Could you check a few things on this model? Use its own coordinates, in mm. Face numbers are marked on the shaded views. A direction names the side the tool comes from. Give positions to 0.01 mm unless a question says otherwise; leave off trailing zeros. Order: outer loops, then holes, each group sorted by start corner. A loop starts at its lowest first (then second) coordinate and runs counter-clockwise, first axis right, second up. Notation, with made-up numbers: M 75.25,-32.5 L 129.25,-32.5 A28 ccw 129.25,2.5 Z; hole C 65,-7.5 d11. An arc over 180 degrees is marked long. Use a Markdown table: item, result. Add a question column.
```python
from build123d import *

# Parameters (mm, degrees)
F0_R          = 5
F1_DEPTH      = 10.1
F2_R          = 4.8
F3_DEPTH      = 3
F5_DEPTH      = 5
F5_DEPTH_BACK = 68
F6_R          = 6
F7_DEPTH      = 3
F8_R          = 5
F9_DEPTH      = 40
F10_R         = 2.5
F11_DEPTH     = 80


with BuildPart() as f1:
    # F0 (on Right) → F1 (new body)
    with BuildSketch(Plane.YZ):
        Circle(F0_R)
    extrude(amount=-F1_DEPTH)

    # F2 (on face) → F3 (join)
    with BuildSketch(Plane.YZ):
        Circle(F2_R)
    extrude(amount=F3_DEPTH)

    # F4 (on face) → F5 (join, two sides)
    with BuildSketch(Plane.YZ.offset(3)) as f5_sk:
        Polygon((-4.565071, -1.483282), (0, -4.8), (4.565071, -1.483282), (2.821369, 3.883282), (-2.821369, 3.883282), align=None)
    extrude(amount=F5_DEPTH)
    extrude(f5_sk.sketch, amount=-F5_DEPTH_BACK)

    # F6 (on face) → F7 (join)
    with BuildSketch(Plane(origin=(-10.1, 0, 0), x_dir=(0, -1, 0), z_dir=(-1, 0, 0))):
        Circle(F6_R)
    extrude(amount=F7_DEPTH)

    # F8 (on face) → F9 (join)
    with BuildSketch(Plane(origin=(-13.1, 0, 0), x_dir=(0, -1, 0), z_dir=(-1, 0, 0))):
        Circle(F8_R)
    extrude(amount=F9_DEPTH)

    # F10 (on face) → F11 (cut)
    with BuildSketch(Plane.YZ.offset(8)):
        Circle(F10_R)
    extrude(amount=-F11_DEPTH, mode=Mode.SUBTRACT)


solid = f1.part
```
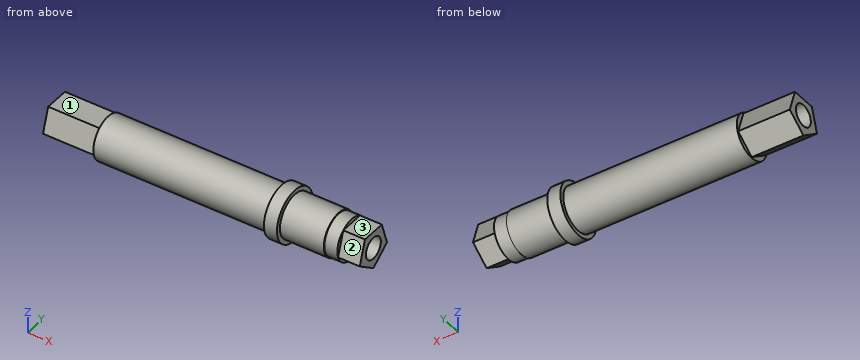
1) For pin 1 (6 mm diameter, centred on x = -44, y = -4, fed in from -Z); pin 2 (3 mm diameter, centred on y = 1.5, z = -1, fed in from +X); pin 3 (1 mm diameter, centred on x = -43, y = 0.5, fed in from -Z); pin 4 (1.5 mm diameter, centred on x = 5, y = -1, fed in from +Z), each with a flat end and sliding along its axis, tell me the tip position at first contact or that it passes through.
2) Please list where these lines run through material, in increasing order: line 1 (Z direction, x = -41.5, y = 0); line 2 (Y direction, x = -18, z = 0.25); line 3 (X direction, y = 4.75, z = 3). Write a range as from..to.
3) For the marked faces 1, 2 and 3, which set-ups out of +Z, -Z, +X, -X, +Y, -Y let a thin tool reach every point of the face, with its end or its side?
4) Suppose I cut it at A-A on z = -0.75. Please give me the cut outline in (x, y), and give its area (3 significant figures).
5) Suppose I cut it at B-B on y = 1.25. Please give me the cut outline in (x, z), and give its area (3 significant figures).
6) Suppose I cut it at D-D on y = -3.5. Please give me the cut outline in (x, z).
7) Suppose I cut it at C-C on x = -45.5. Please give me the cut outline in (y, z), and give its area (3 significant figures).
Values found:
| question | item | result |
|---|---|---|
| 1 | pin 1 | stops at z = -4.9 |
| 1 | pin 2 | stops at x = 8 |
| 1 | pin 3 | stops at z = -5 |
| 1 | pin 4 | stops at z = 3.88 |
| 2 | line 1 | z = -5..-2.5, 2.5..5 |
| 2 | line 2 | y = -4.99..-2.49, 2.49..4.99 |
| 2 | line 3 | x = -13.1..-10.1 |
| 3 | face 1 | +Z, -X, +Y, -Y |
| 3 | face 2 | +Z, +X, -Y |
| 3 | face 3 | +Z, +X, +Y, -Y |
| 4 | outline | M -65,-4.33 L -53.1,-4.33 L -53.1,-4.94 L -13.1,-4.94 L -13.1,-5.95 L -10.1,-5.95 L -10.1,-4.94 L 0,-4.94 L 0,-4.74 L 3,-4.74 L 3,-4.33 L 8,-4.33 L 8,-2.38 L -65,-2.38 Z; M -65,2.38 L 8,2.38 L 8,4.33 L 3,4.33 L 3,4.74 L 0,4.74 L 0,4.94 L -10.1,4.94 L -10.1,5.95 L -13.1,5.95 L -13.1,4.94 L -53.1,4.94 L -53.1,4.33 L -65,4.33 Z |
| 4 | area | 358 mm^2 |
| 5 | outline | M -65,-3.89 L -53.1,-3.89 L -53.1,-4.84 L -13.1,-4.84 L -13.1,-5.87 L -10.1,-5.87 L -10.1,-4.84 L 0,-4.84 L 0,-4.63 L 3,-4.63 L 3,-3.89 L 8,-3.89 L 8,-2.17 L -65,-2.17 Z; M -65,2.17 L 8,2.17 L 8,3.88 L 3,3.88 L 3,4.63 L 0,4.63 L 0,4.84 L -10.1,4.84 L -10.1,5.87 L -13.1,5.87 L -13.1,4.84 L -53.1,4.84 L -53.1,3.88 L -65,3.88 Z |
| 5 | area | 363 mm^2 |
| 6 | outline | M -65,-2.26 L -53.1,-2.26 L -53.1,-3.57 L -13.1,-3.57 L -13.1,-4.87 L -10.1,-4.87 L -10.1,-3.57 L 0,-3.57 L 0,-3.28 L 3,-3.28 L 3,-2.26 L 8,-2.26 L 8,1.79 L 3,1.79 L 3,3.28 L 0,3.28 L 0,3.57 L -10.1,3.57 L -10.1,4.87 L -13.1,4.87 L -13.1,3.57 L -53.1,3.57 L -53.1,1.79 L -65,1.79 Z |
| 7 | outline | C 0,0 d10; hole C 0,0 d5 |
| 7 | area | 58.9 mm^2 |
